Model file for the job. Use its own axes, mm. A direction names the side the tool comes from. Coordinates: 2 decimals unless noted, no trailing zeros. Order: outer loops, then holes, each group sorted by start corner. A loop starts at its lowest first (then second) coordinate and runs counter-clockwise, first axis right, second up. Notation, with made-up numbers: (50, -0.75) - (69, -0.75) arc R29 ccw to (69, 26.25) - close; hole circle Ø11 at (88.5, -9.5). An arc over 180 degrees is marked (long way). Put each result on its own line as item: value. Start each with the question number.
```python
from build123d import *

# Parameters (mm, degrees)
F0_W     = 914.4
F0_H     = 38.1
F0_R     = 5.1562
F1_DEPTH = 4.7625
F2_W     = 914.4
F2_H     = 4.7625
F3_DEPTH = 33.3375
F5_DEPTH = 38.1


with BuildPart() as f1:
    # F0 (on Front) → F1 (new body)
    with BuildSketch(Plane.XZ):
        Rectangle(F0_W, F0_H)
        with Locations((-196.85, -3.175)):
            Circle(F0_R, mode=Mode.SUBTRACT)
        with Locations((196.85, -3.175)):
            Circle(F0_R, mode=Mode.SUBTRACT)
    extrude(amount=F1_DEPTH)

    # F2 (on face) → F3 (join)
    with BuildSketch(Plane.XZ.offset(4.7625)):
        with Locations((0, 16.66875)):
            Rectangle(F2_W, F2_H)
    extrude(amount=F3_DEPTH)

    # F4 (on face) → F5 (cut)
    with BuildSketch(Plane.XY.offset(19.05)):
        Polygon((450.481942, 0), (457.2, -38.1), (457.2, 0), align=None)
        Polygon((-457.2, 0), (-457.2, -38.1), (-450.481942, 0), align=None)
    extrude(amount=-F5_DEPTH, mode=Mode.SUBTRACT)


solid = f1.part
```
Item 1: Flat gauge pins, fed straight in: pin 1 Ø8 at (x, y) = (245.5, -22.5) entering from -Z; pin 2 Ø12 at (x, z) = (196.85, -3.175) entering from -Y. Where does each tip first touch, or does it go through?
Item 2: 3-axis set-ups, long thin cutter, end or side, ignore diameter. For faces 1 (the face through (-6, 0, 0)), 2 (the face through (-6, -4.762, -2)): which of +Z, -Z, +X, -X, +Y, -Y reach the whole face in a straight line?
Item 3: Wall check: line 1 along Z through (x, y) = (-196, -1); line 2 along Z through (x, y) = (196.85, -2.3); line 3 along Z through (x, y) = (142, -10.5). Give the ranges that are in metal, low to high.
Item 4: Slice it at B-B, the plane y = -17. Give the cut face in (x, z).
Item 5: Slice it at A-A, the plane x = -335. Give the cut face in (y, z).
Here are the results:
1. pin 1: stops at z = 14.29
1. pin 2: stops at y = -4.76
2. face 1: +Z, -Z, +X, -X, +Y
2. face 2: -Z, +X, -X, -Y
3. line 1: z = -19.05 to -8.26, 1.91 to 19.05
3. line 2: z = -19.05 to -8.33, 1.98 to 19.05
3. line 3: z = 14.29 to 19.05
4. outline: (-453.48, 14.29) - (453.48, 14.29) - (453.48, 19.05) - (-453.48, 19.05) - close
5. outline: (-38.1, 14.29) - (-4.76, 14.29) - (-4.76, -19.05) - (0, -19.05) - (0, 19.05) - (-38.1, 19.05) - close
